from build123d import *

# Parameters (mm, degrees)
F2_DEPTH = 25
F3_R     = 5
F4_R     = 1.401412
F5_DEPTH = 12.5
F6_R     = 2.473505
F7_DEPTH = 1.901001


with BuildPart() as f2:
    # F0 (on Front) → F2 (new body)
    with BuildSketch(Plane.XZ):
        with BuildLine():
            Line((-50, 0), (0, 0))
            Line((0, 0), (0, 1.900001))
            Line((0, 1.900001), (-50, 1.900001))
            ThreePointArc((-50, 1.900001), (-52.309698, 3.443292), (-51.767766, 6.167766))
            Line((-51.767766, 6.167766), (-33.996891, 23.938641))
            Line((-33.996891, 23.938641), (-35.4336, 25.188939))
            Line((-35.4336, 25.188939), (-53.11127, 7.51127))
            ThreePointArc((-53.11127, 7.51127), (-54.06507, 2.716193), (-50, 0))
        make_face()
    extrude(amount=F2_DEPTH)

    # F3
    f3_edges = [f2.edges().sort_by_distance(p)[0] for p in [
        (-34.715246, -25, 24.56379),
        (-34.715246, 0, 24.56379),
        (0, -25, 0.950001),
        (0, 0, 0.950001),
    ]]
    fillet(f3_edges, radius=F3_R)

    # F4 (on face) → F5 (cut, symmetric)
    with BuildSketch(Plane(origin=(-30.31127, 0, 30.31127), x_dir=(0, -1, 0), z_dir=(-0.707107, 0, 0.707107))):
        with Locations((5, -12.256087)):
            Circle(F4_R)
        with Locations((20.678569, -11.696595)):
            Circle(F4_R)
    extrude(amount=F5_DEPTH, both=True, mode=Mode.SUBTRACT)

    # F6 (on face) → F7 (cut, through all)
    with BuildSketch(Plane.XY.offset(1.900001)):
        with Locations((-42.235214, -15.046177)):
            Circle(F6_R)
    extrude(amount=-F7_DEPTH, mode=Mode.SUBTRACT)


solid = f2.part
Input: part model. Units: mm. Frame: model coordinates. A direction names the side the tool comes from. Give positions to 0.01 mm unless a question says otherwise; leave off trailing zeros. Write each loop counter-clockwise with the first axis right and the second up, starting at its lowest first coordinate (ties: lowest second). Pieces come first, ordered by that corner, then holes. Notation, with made-up numbers: M 64.5,65.5 L 78.5,65.5 A17 ccw 78.5,87.5 Z; hole C -14.75,11 d9. An arc over 180 degrees is marked long. Use one line per item in the form item = value.
1. Mould query, pull axis Y, two halves, no side actions, for faces 1 (the face through (-38.92, -3.89, 20.38)), 2 (the face through (-37, -25, 1)), 3 (the face through (-54.1, -12.3, 2.8)). Classes: released by +Y, released by -Y, zero draft, split by the parting line, or undercut.
Outcome:
face_1 = undercut
face_2 = released by -Y
face_3 = zero draft
2. First-contact query: P1, Ø2, axis at x = -12, y = -14, coming from the -Z side; P2, Ø10, axis at x = -19, y = -18, coming from the +Z side; P3, Ø6.5, axis at x = -42.24, y = -15.05, coming from the +Z side. Flat tips, straight axial feed; report the tip coordinate or a pass-through.
Outcome:
P1 = 0
P2 = 1.9
P3 = 21.63
3. Ray query, L1, parallel to Z at x = -14.5, y = -14.75; L2, parallel to Z at x = -42, y = -4.5; L3, parallel to X at y = -22.25, z = 8. Return the intervals inside material, ascending.
Outcome:
L1 = 0 to 1.9
L2 = 0 to 1.9, 15.94 to 18.62
L3 = -52.62 to -49.94
4. Cut plane D-D on z = 4.25. Return loops of the section in (x, y), and give its area (3 significant figures).
Outcome:
outline = M -54.4,-25 L -52.5,-25 L -52.5,0 L -54.4,0 Z
area = 47.5 mm²
5. Cut plane A-A on y = -8.5. Return loops of the section in (x, z), and give its area (3 significant figures).
Outcome:
outline = M -53.11,7.51 A4.4 ccw -50,0 L 0,0 L 0,1.9 L -50,1.9 A2.5 cw -51.77,6.17 L -34,23.94 L -35.43,25.19 Z
area = 158 mm²
6. Reachability of faces 4 (the face through (-35.794, -1.504, 23.612)), 5 (the face through (-39.876, -14.303, 0.963)), 6 (the face through (-43.007, -12.325, 14.929)) from +Z, -Z, +X, -X, +Y, -Y: full face, straight path, thin tool, end or side. Return the list, or none.
Outcome:
face_4 = +Z, +X, +Y
face_5 = -Z
face_6 = +X, +Y, -Y
7. Cut plane C-C on y = -15.75. Return loops of the section in (x, z).
Outcome:
outline = M -53.11,7.51 A4.4 ccw -50,0 L -44.61,0 L -44.61,1.9 L -50,1.9 A2.5 cw -51.77,6.17 L -34,23.94 L -35.43,25.19 Z; M -39.86,0 L 0,0 L 0,1.9 L -39.86,1.9 Z
8. Cut plane B-B on x = -46. Return loops of the section in (y, z).
Outcome:
outline = M -25,0 L 0,0 L 0,1.9 L -25,1.9 Z; M -25,11.94 L 0,11.94 L 0,14.62 L -25,14.62 Z
